from build123d import *

# Parameters (mm, degrees)
BOSS_EXTRUDE1_DEPTH       = 6.35
F_6_CLEARANCE_HOLE1_D     = 3.6576
F_6_CLEARANCE_HOLE1_DEPTH = 25.4
F_6_CLEARANCE_HOLE1_TIP   = 1.0988539
FILLET1_R                 = 12.7
F_4_CLEARANCE_HOLE1_D     = 2.9464
F_4_CLEARANCE_HOLE1_DEPTH = 25.4
F_4_CLEARANCE_HOLE1_TIP   = 0.885187864
LPATTERN4_COUNT           = 6
LPATTERN4_PITCH           = 25.4
LPATTERN4_COUNT_DIR2      = 7
LPATTERN4_PITCH_DIR2      = 23.622
SKETCH8_W                 = 22
SKETCH8_H                 = 47.6
CUT_EXTRUDE1_DEPTH        = 214.756408018
F_4_CLEARANCE_HOLE3_D     = 2.159


with BuildPart() as part:
    # Sketch1 → Boss-Extrude1 (new body)
    with BuildSketch(Plane(origin=(0, 0, 0), x_dir=(1, 0, 0), z_dir=(0, 1, 0))):
        with BuildLine():
            Line((65.058096917, 37.174573643), (142.24566953, 81.28))
            ThreePointArc((142.24566953, 81.28), (0, 163.83), (-142.24566953, 81.28))
            Line((-142.24566953, 81.28), (-65.058096917, 37.174573643))
            ThreePointArc((-65.058096917, 37.174573643), (0, 74.93), (65.058096917, 37.174573643))
        make_face()
    extrude(amount=BOSS_EXTRUDE1_DEPTH)

    # 6 Clearance Hole1
    with Locations(Plane(origin=(-50.8, 6.35, -125.73), x_dir=(0, 0, 1), z_dir=(0, 1, 0))):
        with Locations((0, 0), (0, 101.6)):
            Hole(F_6_CLEARANCE_HOLE1_D / 2, depth=F_6_CLEARANCE_HOLE1_DEPTH)
            with Locations((0, 0, -(F_6_CLEARANCE_HOLE1_DEPTH + F_6_CLEARANCE_HOLE1_TIP / 2))):  # 118° drill point
                Cone(0, F_6_CLEARANCE_HOLE1_D / 2, F_6_CLEARANCE_HOLE1_TIP, mode=Mode.SUBTRACT)

    # Fillet1
    fillet1_edges = [part.edges().sort_by_distance(p)[0] for p in [
        (142.24566953, 3.175, -81.28),
        (65.058096917, 3.175, -37.174573643),
        (-65.058096917, 3.175, -37.174573643),
        (-142.24566953, 3.175, -81.28),
    ]]
    fillet(fillet1_edges, radius=FILLET1_R)

    # 4 Clearance Hole1
    with Locations(Plane(origin=(0, 6.35, 0), x_dir=(-1, 0, 0), z_dir=(0, 1, 0))):
        with Locations((-34.5, -133.35), (34.5, -133.35)):
            Hole(F_4_CLEARANCE_HOLE1_D / 2, depth=F_4_CLEARANCE_HOLE1_DEPTH)
            with Locations((0, 0, -(F_4_CLEARANCE_HOLE1_DEPTH + F_4_CLEARANCE_HOLE1_TIP / 2))):  # 118° drill point
                Cone(0, F_4_CLEARANCE_HOLE1_D / 2, F_4_CLEARANCE_HOLE1_TIP, mode=Mode.SUBTRACT)

    # Sketch5 → 10 Clearance Hole1 (revolve, cut)
    with BuildSketch(Plane(origin=(-128.255094273, 6.35, -84.874017323), x_dir=(0, 0, 1), z_dir=(1, 0, 0))):
        Polygon((0, 0), (0, 26.895662253), (2.4892, 25.4), (2.4892, 0), align=None)
    f_10_clearance_hole1 = revolve(axis=Axis((-128.255094273, 12.7, -84.874017323), (0, -1, 0)), mode=Mode.SUBTRACT)

    # LPattern4: 10 Clearance Hole1 6 × 7, 28 skipped
    with Locations(*[Vector(0, 0, -1) * (i * LPATTERN4_PITCH) + Vector(0.8667949394357126, 0, 0.49866475007628064) * (j * LPATTERN4_PITCH_DIR2) for i in range(LPATTERN4_COUNT) for j in range(LPATTERN4_COUNT_DIR2) if (i, j) not in ((0, 0), (0, 4), (0, 5), (0, 6), (1, 0), (1, 4), (1, 5), (1, 6), (2, 0), (2, 1), (2, 4), (2, 6), (3, 0), (3, 1), (3, 2), (3, 4), (3, 6), (4, 0), (4, 1), (4, 2), (4, 3), (4, 4), (4, 6), (5, 0), (5, 1), (5, 2), (5, 3), (5, 4), (5, 6))]):
        add(f_10_clearance_hole1, mode=Mode.SUBTRACT)

    # Mirror4: 10 Clearance Hole1 across plane
    add(f_10_clearance_hole1.mirror(Plane(origin=(0, 0, 0), x_dir=(0, 0, 1), z_dir=(1, 0, 0))), mode=Mode.SUBTRACT)

    # Mirror4 copy 1 sketch → Mirror4 copy 1 (revolve, cut)
    with BuildSketch(Plane(origin=(107.779664214, 6.35, -73.094558596), x_dir=(0, 0, 1), z_dir=(-1, 0, 0))):
        Polygon((0, 0), (0, -26.895662253), (2.4892, -25.4), (2.4892, 0), align=None)
    revolve(axis=Axis((107.779664214, 12.7, -73.094558596), (0, 1, 0)), mode=Mode.SUBTRACT)

    # Mirror4 copy 2 sketch → Mirror4 copy 2 (revolve, cut)
    with BuildSketch(Plane(origin=(87.304234155, 6.35, -61.31509987), x_dir=(0, 0, 1), z_dir=(-1, 0, 0))):
        Polygon((0, 0), (0, -26.895662253), (2.4892, -25.4), (2.4892, 0), align=None)
    revolve(axis=Axis((87.304234155, 12.7, -61.31509987), (0, 1, 0)), mode=Mode.SUBTRACT)

    # Mirror4 copy 3 sketch → Mirror4 copy 3 (revolve, cut)
    with BuildSketch(Plane(origin=(66.828804095, 6.35, -49.535641144), x_dir=(0, 0, 1), z_dir=(-1, 0, 0))):
        Polygon((0, 0), (0, -26.895662253), (2.4892, -25.4), (2.4892, 0), align=None)
    revolve(axis=Axis((66.828804095, 12.7, -49.535641144), (0, 1, 0)), mode=Mode.SUBTRACT)

    # Mirror4 copy 4 sketch → Mirror4 copy 4 (revolve, cut)
    with BuildSketch(Plane(origin=(107.779664214, 6.35, -98.494558596), x_dir=(0, 0, 1), z_dir=(-1, 0, 0))):
        Polygon((0, 0), (0, -26.895662253), (2.4892, -25.4), (2.4892, 0), align=None)
    revolve(axis=Axis((107.779664214, 12.7, -98.494558596), (0, 1, 0)), mode=Mode.SUBTRACT)

    # Mirror4 copy 5 sketch → Mirror4 copy 5 (revolve, cut)
    with BuildSketch(Plane(origin=(87.304234155, 6.35, -86.71509987), x_dir=(0, 0, 1), z_dir=(-1, 0, 0))):
        Polygon((0, 0), (0, -26.895662253), (2.4892, -25.4), (2.4892, 0), align=None)
    revolve(axis=Axis((87.304234155, 12.7, -86.71509987), (0, 1, 0)), mode=Mode.SUBTRACT)

    # Mirror4 copy 6 sketch → Mirror4 copy 6 (revolve, cut)
    with BuildSketch(Plane(origin=(66.828804095, 6.35, -74.935641144), x_dir=(0, 0, 1), z_dir=(-1, 0, 0))):
        Polygon((0, 0), (0, -26.895662253), (2.4892, -25.4), (2.4892, 0), align=None)
    revolve(axis=Axis((66.828804095, 12.7, -74.935641144), (0, 1, 0)), mode=Mode.SUBTRACT)

    # Mirror4 copy 7 sketch → Mirror4 copy 7 (revolve, cut)
    with BuildSketch(Plane(origin=(87.304234155, 6.35, -112.11509987), x_dir=(0, 0, 1), z_dir=(-1, 0, 0))):
        Polygon((0, 0), (0, -26.895662253), (2.4892, -25.4), (2.4892, 0), align=None)
    revolve(axis=Axis((87.304234155, 12.7, -112.11509987), (0, 1, 0)), mode=Mode.SUBTRACT)

    # Mirror4 copy 8 sketch → Mirror4 copy 8 (revolve, cut)
    with BuildSketch(Plane(origin=(66.828804095, 6.35, -100.335641144), x_dir=(0, 0, 1), z_dir=(-1, 0, 0))):
        Polygon((0, 0), (0, -26.895662253), (2.4892, -25.4), (2.4892, 0), align=None)
    revolve(axis=Axis((66.828804095, 12.7, -100.335641144), (0, 1, 0)), mode=Mode.SUBTRACT)

    # Mirror4 copy 9 sketch → Mirror4 copy 9 (revolve, cut)
    with BuildSketch(Plane(origin=(25.877943977, 6.35, -76.776723691), x_dir=(0, 0, 1), z_dir=(-1, 0, 0))):
        Polygon((0, 0), (0, -26.895662253), (2.4892, -25.4), (2.4892, 0), align=None)
    revolve(axis=Axis((25.877943977, 12.7, -76.776723691), (0, 1, 0)), mode=Mode.SUBTRACT)

    # Mirror4 copy 10 sketch → Mirror4 copy 10 (revolve, cut)
    with BuildSketch(Plane(origin=(66.828804095, 6.35, -125.735641144), x_dir=(0, 0, 1), z_dir=(-1, 0, 0))):
        Polygon((0, 0), (0, -26.895662253), (2.4892, -25.4), (2.4892, 0), align=None)
    revolve(axis=Axis((66.828804095, 12.7, -125.735641144), (0, 1, 0)), mode=Mode.SUBTRACT)

    # Mirror4 copy 11 sketch → Mirror4 copy 11 (revolve, cut)
    with BuildSketch(Plane(origin=(25.877943977, 6.35, -102.176723691), x_dir=(0, 0, 1), z_dir=(-1, 0, 0))):
        Polygon((0, 0), (0, -26.895662253), (2.4892, -25.4), (2.4892, 0), align=None)
    revolve(axis=Axis((25.877943977, 12.7, -102.176723691), (0, 1, 0)), mode=Mode.SUBTRACT)

    # Mirror4 copy 12 sketch → Mirror4 copy 12 (revolve, cut)
    with BuildSketch(Plane(origin=(25.877943977, 6.35, -127.576723691), x_dir=(0, 0, 1), z_dir=(-1, 0, 0))):
        Polygon((0, 0), (0, -26.895662253), (2.4892, -25.4), (2.4892, 0), align=None)
    revolve(axis=Axis((25.877943977, 12.7, -127.576723691), (0, 1, 0)), mode=Mode.SUBTRACT)

    # Mirror4 copy 13 sketch → Mirror4 copy 13 (revolve, cut)
    with BuildSketch(Plane(origin=(25.877943977, 6.35, -152.976723691), x_dir=(0, 0, 1), z_dir=(-1, 0, 0))):
        Polygon((0, 0), (0, -26.895662253), (2.4892, -25.4), (2.4892, 0), align=None)
    revolve(axis=Axis((25.877943977, 12.7, -152.976723691), (0, 1, 0)), mode=Mode.SUBTRACT)

    # Sketch8 → Cut-Extrude1 (cut, through all)
    with BuildSketch(Plane(origin=(0, 6.35, 0), x_dir=(1, 0, 0), z_dir=(0, 1, 0))):
        with Locations((0, 119.38)):
            Rectangle(SKETCH8_W, SKETCH8_H)
    extrude(amount=-CUT_EXTRUDE1_DEPTH, mode=Mode.SUBTRACT)

    # 4 Clearance Hole3 (through all)
    with Locations(Plane(origin=(0, 6.35, 0), x_dir=(-1, 0, 0), z_dir=(0, 1, 0))):
        with Locations((13.4, -125.08), (13.4, -117.08), (13.4, -109.08), (13.4, -101.08), (-13.4, -101.08), (-13.4, -109.08), (-13.4, -117.08), (-13.4, -125.08)):
            Hole(F_4_CLEARANCE_HOLE3_D / 2)


solid = part.part
Can you work these out from the model? Positions are in its coordinate system, mm. A direction names the side the tool comes from. Round coordinates to 2 decimals unless told otherwise and drop trailing zeros. Write each question's results on one line, items separated by ' | '. Start each with the question number.
1) Which directions (+Z, -Z, +X, -X, +Y, -Y) give clear straight access to the entire face, cutting with the end or side of a thin tool? Please do faces 4 (the flat face through (-103.41, 3.13, -59.09)), 5 (the flat face through (-11, 3, -119)).
2) For pin 1 Ø3 at (x, y) = (-49, 1) entering from -Z; pin 2 Ø2 at (y, z) = (3, -80) entering from +X; pin 3 Ø3 at (x, y) = (-37.5, 4.5) entering from -Z, each with a flat end and sliding along its axis, tell me the tip position at first contact or that it passes through.
3) We'd pull the mould along X, two halves only. Please class faces 1 (the flat face through (102.63, 3.131, -58.643)), 2 (the flat face through (-2, 6.35, -90)), 3 (the cylindrical face through (126.74, 3.22, -86.85)): released by +X, released by -X, zero draft, split by the parting line, or undercut.
4) Suppose I cut it at A-A (y = 3.75). Give the number of separate pieces and of enclosed holes in the cut face, and give its area (3 significant figures).
5) Please list where these lines run through material, in increasing order: line 1 (Z direction, x = 13.5, y = 5.5); line 2 (X direction, y = 6.25, z = -151); line 3 (X direction, y = 5.25, z = -117.08).
Here are the results:
1) face 4: +Z, -X, +Y, -Y | face 5: +Y, -Y
2) pin 1: stops at z = -156.79 | pin 2: stops at x = 136.24 | pin 3: stops at z = -159.83
3) face 1: released by +X | face 2: zero draft | face 3: undercut
4) separate pieces: 1 | enclosed holes: 41 | area: 20,500 mm2
5) line 1: z = -163.27 to -126.15, -124.01 to -118.15, -116.01 to -110.15, -108.01 to -102.15, -100.01 to -73.7 | line 2: x = -63.56 to -27.39, -24.37 to 24.37, 27.39 to 63.56 | line 3: x = -114.6 to -14.48, -12.32 to -11, 11 to 12.32, 14.48 to 114.6
